Drawing for the job (mm, zero at the part's lowest x, y, z). Round coordinates to 2 decimals unless told otherwise and drop trailing zeros. Loops run counter-clockwise (first coordinate to the right, second up) from the corner with the lowest first, then second, coordinate; pieces in that order, holes last. Notation, with made-up numbers: (-19, 59) -> (33, 59) arc R37 cw to (33, 98) -> close; hole circle Ø10 at (68.25, 26). An arc over 180 degrees is marked (long way). Put each result on its own line as item: value. Start each with the question number.
Item 1: Cut at B-B, the plane x = 3.25. Count the separate pieces of the cut face and the enclosed holes in it, plus the area to 3 significant figures.
Item 2: Cut at A-A, the plane y = 12.7. List the corners of the cut face in (x, z).
Item 3: Drill centre lines: probe 1 along Z at (x, y) = (4.5, 32); probe 2 along Z at (x, y) = (3, 109.5) (1 decimal). Where is each one in solid material? Low to high. Write a range as [from, to].
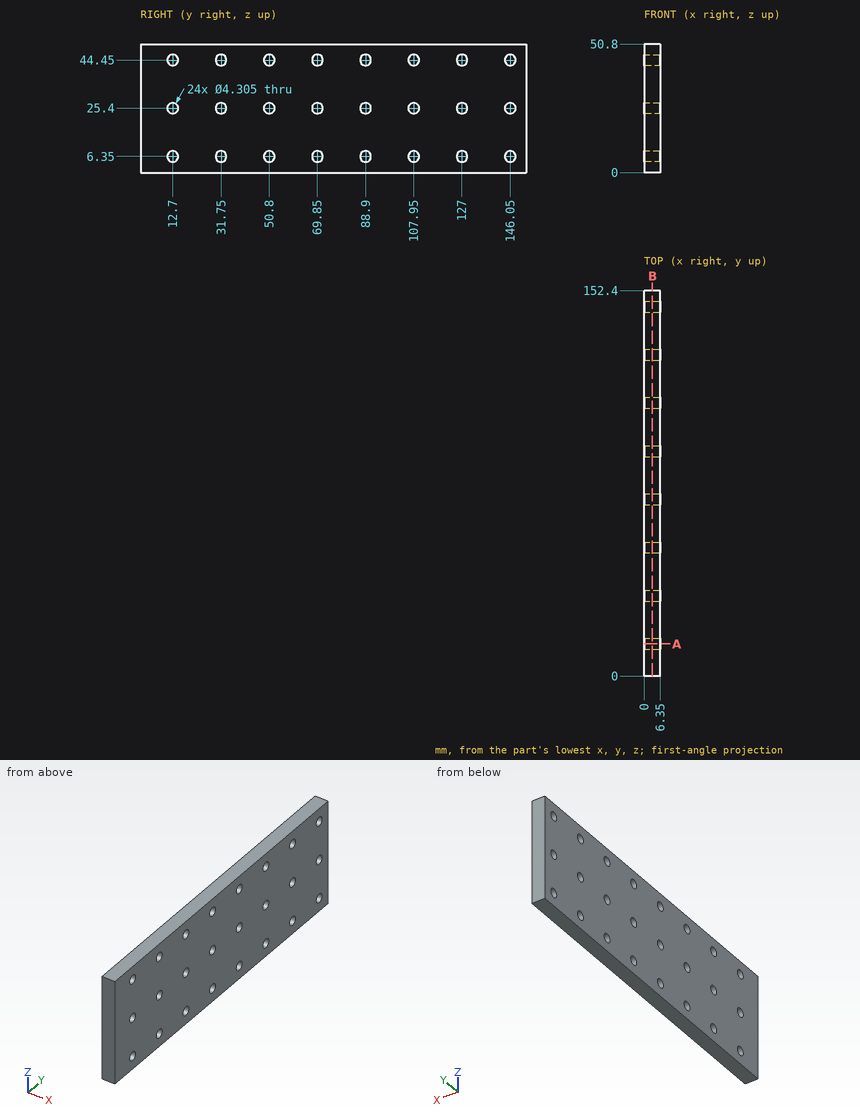
Reply:
1. separate pieces: 1
1. enclosed holes: 24
1. area: 7,390 mm^2
2. outline: (0, 0) -> (6.35, 0) -> (6.35, 4.2) -> (0, 4.2) -> close; (0, 8.5) -> (6.35, 8.5) -> (6.35, 23.25) -> (0, 23.25) -> close; (0, 27.55) -> (6.35, 27.55) -> (6.35, 42.3) -> (0, 42.3) -> close; (0, 46.6) -> (6.35, 46.6) -> (6.35, 50.8) -> (0, 50.8) -> close
3. probe 1: z = [0, 4.21], [8.49, 23.26], [27.54, 42.31], [46.59, 50.8]
3. probe 2: z = [0, 4.9], [7.8, 23.9], [26.9, 43], [45.9, 50.8]
